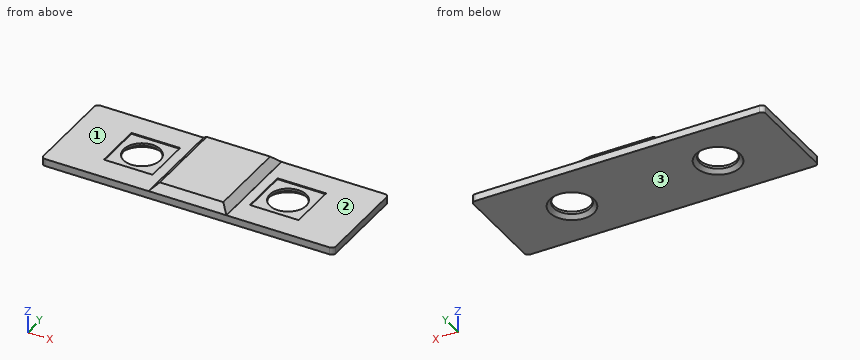
from build123d import *

# Parameters (mm, degrees)
SKETCH_W        = 76.2
SKETCH_H        = 25.4
SKETCH_R        = 4.7625
PAD_DEPTH       = 1.905
SKETCH001_W     = 12.7
SKETCH001_H     = 12.7
POCKET_DEPTH    = 0.254
CHAMFER_SIZE    = 1
FILLET_R        = 1
SKETCH002_W     = 20.32
SKETCH002_H     = 25.4
PAD001_DEPTH    = 1.905
CHAMFER001_SIZE = 1.889001


with BuildPart() as part:
    # Sketch → Pad (new body)
    with BuildSketch(Plane.XY):
        Rectangle(SKETCH_W, SKETCH_H)
        with Locations((-19.05, 0)):
            Circle(SKETCH_R, mode=Mode.SUBTRACT)
        with Locations((19.05, 0)):
            Circle(SKETCH_R, mode=Mode.SUBTRACT)
    extrude(amount=PAD_DEPTH)

    # Sketch001 → Pocket (cut)
    with BuildSketch(Plane.XY.offset(1.905)):
        with Locations((-19.05, 0)):
            Rectangle(SKETCH001_W, SKETCH001_H)
        with Locations((19.05, 0)):
            Rectangle(SKETCH001_W, SKETCH001_H)
    extrude(amount=-POCKET_DEPTH, mode=Mode.SUBTRACT)

    # Chamfer
    chamfer_edges = [part.edges().sort_by_distance(p)[0] for p in [
        (14.2875, 0, 0),
        (-23.8125, 0, 0),
    ]]
    chamfer(chamfer_edges, length=CHAMFER_SIZE)

    # Fillet
    fillet_edges = [part.edges().sort_by_distance(p)[0] for p in [
        (38.1, 12.7, 0.9525),
        (38.1, -12.7, 0.9525),
        (-38.1, -12.7, 0.9525),
        (-38.1, 12.7, 0.9525),
    ]]
    fillet(fillet_edges, radius=FILLET_R)

    # Sketch002 (on Face5 of Pocket) → Pad001 (join)
    with BuildSketch(Plane.XY.offset(1.905)):
        Rectangle(SKETCH002_W, SKETCH002_H)
    extrude(amount=PAD001_DEPTH)

    # Chamfer001
    chamfer001_edges = [part.edges().sort_by_distance(p)[0] for p in [
        (0, -12.7, 3.81),
        (-10.16, 0, 3.81),
        (10.16, 0, 3.81),
        (0, 12.7, 3.81),
    ]]
    chamfer(chamfer001_edges, length=CHAMFER001_SIZE)


solid = part.part
Source: CAD feature listing. Evaluate the final solid. Frame: model axes, mm. Face numbers are marked on the shaded views. A direction names the side the tool comes from. Round coordinates to 2 decimals unless told otherwise and drop trailing zeros. Loops run counter-clockwise (first coordinate to the right, second up) from the corner with the lowest first, then second, coordinate; pieces in that order, holes last.
Q1. First-contact query: P1, Ø14, axis at x = 17.5, y = -2, coming from the +Z side (3 decimals); P2, Ø1.5, axis at y = 0, z = 3, coming from the +X side; P3, Ø7.5, axis at x = -19.05, y = 0, coming from the -Z side. Flat tips, straight axial feed; report the tip coordinate or a pass-through.
Q2. Ray query, line 1 (X direction, y = 0, z = 1.3); line 2 (Y direction, x = 19.05, z = 1.45); line 3 (Z direction, x = 25, y = -9.25) (3 decimals). Return the intervals inside material, ascending.
Q3. Access query for the marked faces 1, 2 and 3. Directions: +Z, -Z, +X, -X, +Y, -Y. A direction counts if a zero-diameter tool reaches every point of the face in a straight line with its end or side. Return the directions, or none.
Q4. Section C-C, the plane x = -3. Return loops of the section in (y, z).
Q5. Section B-B, the plane y = 0. State how many separate pieces and enclosed holes the cut face has, plus the area to 3 significant figures.
Q6. Section D-D, the plane y = 8. Return loops of the section in (x, z) (3 decimals), plus the area to 3 significant figures.
Solutions:
1. P1: stops at z = 1.905
1. P2: stops at x = 9.83
1. P3: passes through
2. line 1: x = -38.1 to -23.81, -14.29 to 14.29, 23.81 to 38.1
2. line 2: y = -12.7 to -4.76, 4.76 to 12.7
2. line 3: z = 0 to 1.905
3. face 1: +Z, -X, +Y, -Y
3. face 2: +Z, +X, +Y, -Y
3. face 3: -Z, +X, -X, +Y, -Y
4. outline: (-12.7, 0) - (12.7, 0) - (12.7, 1.92) - (10.81, 3.81) - (-10.81, 3.81) - (-12.7, 1.92) - close
5. separate pieces: 3
5. enclosed holes: 0
5. area: 140 mm2
6. outline: (-38.1, 0) - (38.1, 0) - (38.1, 1.905) - (10.16, 1.905) - (10.16, 1.921) - (8.271, 3.81) - (-8.271, 3.81) - (-10.16, 1.921) - (-10.16, 1.905) - (-38.1, 1.905) - close
6. area: 180 mm2
